The model under review builds one solid part; all positions refer to its coordinate system, in mm. A direction names the side the tool comes from. Coordinates: 2 decimals unless noted, no trailing zeros. Loops run counter-clockwise (first coordinate to the right, second up) from the corner with the lowest first, then second, coordinate; pieces in that order, holes last. Notation, with made-up numbers: (73, -1.5) - (112, -1.5) arc R21 cw to (112, 19.5) - close; hole circle Ø2 at (15, 67). An arc over 180 degrees is marked (long way). Answer in a Markdown table with one row per item. Add a question column.
(1) For P1, Ø5.5, axis at x = 0, y = 0, coming from the +Z side; P2, Ø12, axis at y = -28.5, z = 38, coming from the +X side; P3, Ø6, axis at y = 21, z = 38.5, coming from the -X side; P4, Ø3, axis at y = -34, z = 52.5, coming from the +X side, all flat-tipped, find the tip position at first contact; note any pin that passes through.
(2) We need section B-B on z = 36. Give the number of separate pieces and of enclosed holes in the cut face, plus the area to 3 significant figures.
(3) For line 1 along X through (y, z) = (1, 30.5); line 2 along Y through (x, z) = (0, 3); line 3 along X through (y, z) = (3, 30), list the stretches that pass through material, from the lowest coordinate up.
(4) We need section A-A on y = 0. Write out the cut boundary in (x, z), plus the area to 3 significant figures.
(5) Machinability: for faces 5 (the flat face through (-16.987, -34, 33)), 6 (the cylindrical face through (-5.4, -24.28, 34.58)), 7 (the cylindrical face through (-32.64, 2.67, 32.04)), which of the approach directions +Z, -Z, +X, -X, +Y, -Y give a long, thin tool a straight path to every point of the face, cutting with its end or side? Answer none if there is none.
(6) Mouldability with a two-part tool opening along X and no side actions: class faces 1 (the flat face through (16.987, -34, 33)), 2 (the flat face through (30.75, 0, 35)), 3 (the flat face through (7, -5, 0)), 4 (the flat face through (17, -20, 5)) as +X half, -X half, draft (parallel to the pull), parting line (faces both ways), or undercut.
from build123d import *

# Parameters (mm, degrees)
SKETCH2_R                       = 4.79
BOSS_EXTRUDE2_DEPTH             = 65
SHELL4_START                    = 5
SHELL4_OUTLINE_R                = 4.79
SHELL4_DEPTH                    = 60
SKETCH3_W                       = 33.974254958
SKETCH3_H                       = 12
BOSS_EXTRUDE3_DEPTH             = 65
SKETCH4_W                       = 14.974254958
SKETCH4_H                       = 4
CUT_EXTRUDE1_DEPTH              = 30
BOSS_EXTRUDE4_DEPTH             = 60
CIRPATTERN2_COUNT               = 3
CIRPATTERN2_ANGLE               = 50
CIRPATTERN2_THE_OTHER_WAY_COUNT = 3
CIRPATTERN2_THE_OTHER_WAY_ANGLE = 50
SKETCH5_4_W                     = 9.6
SKETCH5_4_H                     = 9.8
CUT_EXTRUDE2_DEPTH              = 60
CIRPATTERN3_COUNT               = 2
CIRPATTERN3_ANGLE               = 50
CIRPATTERN3_THE_OTHER_WAY_COUNT = 2
CIRPATTERN3_THE_OTHER_WAY_ANGLE = 50
MIRROR1_START                   = 5
MIRROR1_DEPTH                   = 60
MIRROR1_2_DEPTH                 = 60
FILLET2_R                       = 10
FILLET6_R                       = 7


# Read off the part's stored shape, not the designer's step: Shell4, Mirror1
with BuildPart() as part:
    # Sketch2 → Boss-Extrude2 (new body)
    with BuildSketch(Plane.XY):
        with BuildLine():
            Line((13.136304655, 30), (-13.136304655, 30))
            ThreePointArc((-13.136304655, 30), (-32.678055188, 2.169610358), (-16.987127479, -28))
            Line((-16.987127479, -28), (16.987127479, -28))
            ThreePointArc((16.987127479, -28), (32.678055188, 2.169610358), (13.136304655, 30))
        make_face()
        Circle(SKETCH2_R, mode=Mode.SUBTRACT)
    extrude(amount=BOSS_EXTRUDE2_DEPTH)

    # Shell4 outline → Shell4 (cut)
    with BuildSketch(Plane.XY.offset(SHELL4_START)):
        with BuildLine():
            ThreePointArc((-12.710723819, 28), (-30.677774708, 2.106333062), (-16.418358627, -26))
            Line((-16.418358627, -26), (16.418358627, -26))
            ThreePointArc((16.418358627, -26), (30.677774708, 2.106333062), (12.710723819, 28))
            Line((12.710723819, 28), (-12.710723819, 28))
        make_face()
        Circle(SHELL4_OUTLINE_R, mode=Mode.SUBTRACT)
    extrude(amount=SHELL4_DEPTH, mode=Mode.SUBTRACT)

    # Sketch3 → Boss-Extrude3 (add)
    with BuildSketch(Plane.XY.offset(65)):
        with Locations((0, -34)):
            Rectangle(SKETCH3_W, SKETCH3_H)
    extrude(amount=-BOSS_EXTRUDE3_DEPTH)

    # Sketch4 → Cut-Extrude1 (cut)
    with BuildSketch(Plane.XY.offset(65)):
        with Locations((0, -34)):
            Rectangle(SKETCH4_W, SKETCH4_H)
    extrude(amount=-CUT_EXTRUDE1_DEPTH, mode=Mode.SUBTRACT)

    # Sketch5 → Boss-Extrude4 (add)
    with BuildSketch(Plane.XY.offset(5)):
        with BuildLine():
            Line((21.15, 0), (20.35, 0))
            Line((20.35, 0), (20.35, -7))
            Line((20.35, -7), (29.551861194, -8.5))
            ThreePointArc((29.551861194, -8.5), (30.008505534, -6.712085787), (30.357083193, -4.9))
            Line((30.357083193, -4.9), (21.15, -4.9))
            Line((21.15, -4.9), (21.15, 0))
        make_face()
        with BuildLine():
            Line((20.35, 7), (20.35, 0))
            Line((20.35, 0), (21.15, 0))
            Line((21.15, 0), (21.15, 4.9))
            Line((21.15, 4.9), (30.357083193, 4.9))
            ThreePointArc((30.357083193, 4.9), (30.008505534, 6.712085787), (29.551861194, 8.5))
            Line((29.551861194, 8.5), (20.35, 7))
        make_face()
        with BuildLine():
            Line((30.75, 0), (21.15, 0))
            Line((21.15, 0), (21.15, -4.9))
            Line((21.15, -4.9), (30.357083193, -4.9))
            ThreePointArc((30.357083193, -4.9), (30.651613401, -2.457864094), (30.75, 0))
        make_face()
        with BuildLine():
            Line((21.15, 4.9), (21.15, 0))
            Line((21.15, 0), (30.75, 0))
            ThreePointArc((30.75, 0), (30.651613401, 2.457864094), (30.357083193, 4.9))
            Line((30.357083193, 4.9), (21.15, 4.9))
        make_face()
    boss_extrude4 = extrude(amount=BOSS_EXTRUDE4_DEPTH)

    # CirPattern2: Boss-Extrude4 ×3 about axis
    cirpattern2_axis = Axis((0, 0, 0), (0, 0, -1))
    for i in range(1, CIRPATTERN2_COUNT):
        add(boss_extrude4.rotate(cirpattern2_axis, i * CIRPATTERN2_ANGLE / (CIRPATTERN2_COUNT - 1)))

    # CirPattern2 the other way: Boss-Extrude4 ×3 about axis
    cirpattern2_the_other_way_axis = Axis((0, 0, 0), (0, 0, 1))
    for i in range(1, CIRPATTERN2_THE_OTHER_WAY_COUNT):
        add(boss_extrude4.rotate(cirpattern2_the_other_way_axis, i * CIRPATTERN2_THE_OTHER_WAY_ANGLE / (CIRPATTERN2_THE_OTHER_WAY_COUNT - 1)))

    # Sketch5<4> → Cut-Extrude2 (cut)
    with BuildSketch(Plane.XY.offset(5)):
        with Locations((25.95, 0)):
            Rectangle(SKETCH5_4_W, SKETCH5_4_H)
    cut_extrude2 = extrude(amount=CUT_EXTRUDE2_DEPTH, mode=Mode.SUBTRACT)

    # CirPattern3: Cut-Extrude2 ×2 about axis
    cirpattern3_axis = Axis((0, 0, 0), (0, 0, 1))
    for i in range(1, CIRPATTERN3_COUNT):
        add(cut_extrude2.rotate(cirpattern3_axis, i * CIRPATTERN3_ANGLE / (CIRPATTERN3_COUNT - 1)), mode=Mode.SUBTRACT)

    # CirPattern3 the other way: Cut-Extrude2 ×2 about axis
    cirpattern3_the_other_way_axis = Axis((0, 0, 0), (0, 0, -1))
    for i in range(1, CIRPATTERN3_THE_OTHER_WAY_COUNT):
        add(cut_extrude2.rotate(cirpattern3_the_other_way_axis, i * CIRPATTERN3_THE_OTHER_WAY_ANGLE / (CIRPATTERN3_THE_OTHER_WAY_COUNT - 1)), mode=Mode.SUBTRACT)

    # Mirror1 outline → Mirror1 (cut)
    with BuildSketch(Plane.XY.offset(MIRROR1_START)):
        with BuildLine():
            Line((-30.357083193, 4.9), (-30.75, 4.9))
            Line((-30.75, 4.9), (-30.75, 0))
            ThreePointArc((-30.75, 0), (-30.651613401, 2.457864094), (-30.357083193, 4.9))
        make_face()
        with BuildLine():
            ThreePointArc((-30.357083193, -4.9), (-30.651613401, -2.457864094), (-30.75, 0))
            Line((-30.75, 0), (-30.75, -4.9))
            Line((-30.75, -4.9), (-30.357083193, -4.9))
        make_face()
        with BuildLine():
            Line((-23.519336769, 20.406207338), (-23.266774714, 20.105215602))
            ThreePointArc((-23.266774714, 20.105215602), (-21.585264808, 21.90065851), (-19.765620831, 23.555948998))
            Line((-19.765620831, 23.555948998), (-23.519336769, 20.406207338))
        make_face()
        with BuildLine():
            Line((-16.012101227, 26.705525913), (-19.765620831, 23.555948998))
            ThreePointArc((-19.765620831, 23.555948998), (-17.819591962, 25.060419835), (-15.759539172, 26.404534177))
            Line((-15.759539172, 26.404534177), (-16.012101227, 26.705525913))
        make_face()
        with BuildLine():
            ThreePointArc((-19.765615493, -23.555953477), (-21.585262326, -21.900660956), (-23.266774714, -20.105215602))
            Line((-23.266774714, -20.105215602), (-23.519336769, -20.406207338))
            Line((-23.519336769, -20.406207338), (-19.765615493, -23.555953477))
        make_face()
        with BuildLine():
            ThreePointArc((-16.418358627, -26), (-18.133210875, -24.834435032), (-19.765615493, -23.555953477))
            Line((-19.765615493, -23.555953477), (-16.012101227, -26.705525913))
            Line((-16.012101227, -26.705525913), (-15.420094694, -26))
            Line((-15.420094694, -26), (-16.418358627, -26))
        make_face()
    extrude(amount=MIRROR1_DEPTH, mode=Mode.SUBTRACT)

    # Mirror1 2 outline → Mirror1 2 (add)
    with BuildSketch(Plane.XY.offset(MIRROR1_START)):
        with BuildLine():
            ThreePointArc((-23.266774714, 20.105215602), (-27.868964451, 12.995511548), (-30.357083193, 4.9))
            Line((-30.357083193, 4.9), (-21.15, 4.9))
            Line((-21.15, 4.9), (-21.15, -4.9))
            Line((-21.15, -4.9), (-30.357083193, -4.9))
            ThreePointArc((-30.357083193, -4.9), (-27.868964451, -12.995511548), (-23.266774714, -20.105215602))
            Line((-23.266774714, -20.105215602), (-17.348575716, -13.052180685))
            Line((-17.348575716, -13.052180685), (-9.841340174, -19.351499259))
            Line((-9.841340174, -19.351499259), (-15.420094694, -26))
            Line((-15.420094694, -26), (-11.234208489, -26))
            Line((-11.234208489, -26), (-7.718416755, -20.088517685))
            Line((-7.718416755, -20.088517685), (-16.536726932, -12.689076868))
            Line((-16.536726932, -12.689076868), (-20.35, -4.511486385))
            Line((-20.35, -4.511486385), (-20.35, 4.511486385))
            Line((-20.35, 4.511486385), (-16.536726932, 12.689076868))
            Line((-16.536726932, 12.689076868), (-7.718416755, 20.088517685))
            Line((-7.718416755, 20.088517685), (-12.423687387, 28))
            Line((-12.423687387, 28), (-12.710723819, 28))
            ThreePointArc((-12.710723819, 28), (-14.257466342, 27.244947302), (-15.759539172, 26.404534177))
            Line((-15.759539172, 26.404534177), (-9.841340174, 19.351499259))
            Line((-9.841340174, 19.351499259), (-17.348575716, 13.052180685))
            Line((-17.348575716, 13.052180685), (-23.266774714, 20.105215602))
        make_face()
    extrude(amount=MIRROR1_2_DEPTH)

    # Fillet2
    fillet2_edges = [part.edges().sort_by_distance(p)[0] for p in [
        (20.35, 4.511486385, 35),
        (16.536726932, 12.689076868, 35),
        (-20.35, -4.511486385, 35),
        (-16.536726932, -12.689076868, 35),
        (-20.35, 4.511486385, 35),
        (-16.536726932, 12.689076868, 35),
        (20.35, -4.511486385, 35),
        (16.536726932, -12.689076868, 35),
    ]]
    fillet(fillet2_edges, radius=FILLET2_R)

    # Fillet6
    # the kernel refuses this fillet: 7 mm, written as the material it adds along each edge
    with BuildSketch(Plane(origin=(12.423687387, 28, 5), x_dir=(-0.5111673704735938, -0.8594811919775275, 0), z_dir=(0, 0, 1))) as fillet6_piece_1:
        with BuildLine():
            CenterArc((11.96925694, -6.431066244), FILLET6_R, 113.259789789, 97.48182924)
            Line((5.952888596, -10.009237838), (5.832561229, -10.08080127))
            Line((5.832561229, -10.08080127), (-0.120327367, -0.071563432))
            Line((-0.120327367, -0.071563432), (0, 0.14))
            ThreePointArc((0, 0.14), (4.602475533, 0.14), (9.149664949, 0.128621325))
            Line((9.149664949, 0.128621325), (9.204951066, 0))
        make_face()
    extrude(amount=60)
    with BuildSketch(Plane(origin=(-11.234208489, -26, 5), x_dir=(1, 0, 0), z_dir=(0, 0, 1))) as fillet6_piece_2:
        with BuildLine():
            CenterArc((10.430640196, 7), FILLET6_R, 188.945942292, 81.054057708)
            Line((3.515791734, 5.911482315), (3.377494765, 5.889711961))
            ThreePointArc((3.377494765, 5.889711961), (1.6375685, 3.027304589), (-0.120327367, 0.071563432))
            Line((-0.120327367, 0.071563432), (0, -0.14))
            Line((0, -0.14), (10.430640196, -0.14))
            Line((10.430640196, -0.14), (10.430640196, 0))
        make_face()
    extrude(amount=60)
    with BuildSketch(Plane(origin=(-12.423687387, 28, 5), x_dir=(1, 0, 0), z_dir=(0, 0, 1))) as fillet6_piece_3:
        with BuildLine():
            CenterArc((11.645674078, -7), FILLET6_R, 90, 97.481829242)
            Line((4.705270632, -7.911482315), (4.566462563, -7.929711961))
            ThreePointArc((4.566462563, -7.929711961), (2.232307949, -4.027304589), (-0.120327367, -0.071563432))
            Line((-0.120327367, -0.071563432), (0, 0.14))
            Line((0, 0.14), (11.645674078, 0.14))
            Line((11.645674078, 0.14), (11.645674078, 0))
        make_face()
    extrude(amount=60)
    with BuildSketch(Plane(origin=(11.234208489, -26, 65), x_dir=(-0.5111673704735934, 0.8594811919775279, 0), z_dir=(0, 0, -1))) as fillet6_piece_4:
        with BuildLine():
            CenterArc((11.348171265, -5.386767475), FILLET6_R, 129.687561323, 81.054057706)
            Line((5.331802921, -8.964939069), (5.211475554, -9.036502501))
            Line((5.211475554, -9.036502501), (-0.120327367, -0.071563432))
            Line((-0.120327367, -0.071563432), (0, 0.14))
            ThreePointArc((0, 0.14), (3.438982941, 0.14), (6.788561774, 0.10773535))
            Line((6.788561774, 0.10773535), (6.877965882, 0))
        make_face()
    extrude(amount=60)


solid = part.part
Outcome:
| question | item | result |
|---|---|---|
| 1 | P1 | through |
| 1 | P2 | x = 23.8 |
| 1 | P3 | x = -27.36 |
| 1 | P4 | x = 16.99 |
| 2 | separate pieces | 1 |
| 2 | enclosed holes | 8 |
| 2 | area | 1,500 mm² |
| 3 | line 1 | -32.73 to -30.75, -21.15 to -20.35, 20.35 to 21.15, 30.75 to 32.73 |
| 3 | line 2 | -40 to -4.79, 4.79 to 30 |
| 3 | line 3 | -32.61 to -30.75, -21.15 to -20.33, 20.33 to 21.15, 30.75 to 32.61 |
| 4 | outline | (-32.75, 0) - (-4.79, 0) - (-4.79, 5) - (-20.35, 5) - (-20.35, 65) - (-21.15, 65) - (-21.15, 5) - (-30.75, 5) - (-30.75, 65) - (-32.75, 65) - close; (4.79, 0) - (32.75, 0) - (32.75, 65) - (30.75, 65) - (30.75, 5) - (21.15, 5) - (21.15, 65) - (20.35, 65) - (20.35, 5) - (4.79, 5) - close |
| 4 | area | 616 mm² |
| 5 | face 5 | +Z, -Z, -X, -Y |
| 5 | face 6 | +Z |
| 5 | face 7 | +Z, -Z, -X |
| 6 | face 1 | +X half |
| 6 | face 2 | undercut |
| 6 | face 3 | draft |
| 6 | face 4 | undercut |
